```python
from build123d import *

# Parameters (mm, degrees)
SKETCH_R     = 2
PAD_DEPTH    = 10
PAD001_DEPTH = 10
PAD002_DEPTH = 10


with BuildPart() as part:
    # Sketch → Pad (new body)
    with BuildSketch(Plane.XY):
        with BuildLine():
            Line((-5, -25), (-5, 0))
            ThreePointArc((5, 0), (0, 5), (-5, 0))
            Line((5, 0), (5, -15))
            Line((5, -15), (70, -15))
            Line((70, -15), (70, 0))
            ThreePointArc((80, 0), (75, 5), (70, 0))
            Line((80, 0), (80, -25))
            Line((-5, -25), (80, -25))
        make_face()
        Circle(SKETCH_R, mode=Mode.SUBTRACT)
        with Locations((75, 0)):
            Circle(SKETCH_R, mode=Mode.SUBTRACT)
    extrude(amount=PAD_DEPTH)

    # Sketch001 (on Face1 of Pad) → Pad001 (join)
    with BuildSketch(Plane(origin=(-5, 0, 0), x_dir=(0, -1, 0), z_dir=(-1, 0, 0))):
        Polygon((25, 10), (-5, 61.961524), (-13.660254, 56.961524), (13.452995, 10), align=None)
    extrude(amount=-PAD001_DEPTH)

    # Sketch002 (on Face7 of Pad) → Pad002 (join)
    with BuildSketch(Plane.YZ.offset(80)):
        Polygon((-25, 10), (5, 61.961524), (13.660254, 56.961524), (-13.452995, 10), align=None)
    extrude(amount=-PAD002_DEPTH)


solid = part.part
```
The model under review builds one solid part; all positions refer to its coordinate system, in mm. A direction names the side the tool comes from. Round coordinates to 2 decimals unless told otherwise and drop trailing zeros. Order: outer loops, then holes, each group sorted by start corner. A loop starts at its lowest first (then second) coordinate and runs counter-clockwise, first axis right, second up. Notation, with made-up numbers: M -35.75,58 L 11.25,58 A15 ccw 11.25,86 Z; hole C 16,-39.75 d2. An arc over 180 degrees is marked long. Use a Markdown table: item, result.
1) Draft analysis for pull direction X (two halves, no side actions). For faces 6 (the face through (80, -7, 27)), 7 (the face through (5, -7, 29)), 8 (the face through (-0.07, -10.21, 35.62)), state which applies: released by +X, released by -X, zero draft, split by the parting line, or undercut.
Report:
| item | result |
|---|---|
| face 6 | released by +X |
| face 7 | undercut |
| face 8 | zero draft |
2) Consider section A-A (x = 75). Write out the cut boundary in (y, z), then the cut area to 3 significant figures.
Report:
| item | result |
|---|---|
| outline | M -25,0 L -2,0 L -2,10 L -13.45,10 L 13.66,56.96 L 5,61.96 L -25,10 Z; M 2,0 L 5,0 L 5,10 L 2,10 Z |
| area | 831 mm^2 |
3) Tool access review of faces 1 (the face through (70, -7, 29)), 2 (the face through (75.07, 0.293, 33.809)), 3 (the face through (38, -20, 10)), 4 (the face through (0, 5, 5)), 5 (the face through (37, -15, 5)): name each direction out of +Z, -Z, +X, -X, +Y, -Y from which nothing blocks a thin tool from reaching the whole face with its end or side.
Report:
| item | result |
|---|---|
| face 1 | +Z, +Y |
| face 2 | +X, -X, +Y |
| face 3 | +Z, +Y, -Y |
| face 4 | -Z, +Y |
| face 5 | +Z, -Z, +Y |
4) Insertion check: pin 1 (5 mm diameter, centred on x = 52.5, z = 4, fed in from +Y); pin 2 (8 mm diameter, centred on y = 7.5, z = 12, fed in from -X); pin 3 (2.5 mm diameter, centred on x = 0, y = 0, fed in from +Z). Each pin has a flat end and moves straight along its axis. Give the tip position at first contact, or say it passes through.
Report:
| item | result |
|---|---|
| pin 1 | y = -15 |
| pin 2 | x = -2.95 |
| pin 3 | z = 55.47 |
5) Consider section C-C (y = 8). Write out the cut boundary in (x, z), then the cut area to 3 significant figures.
Report:
| item | result |
|---|---|
| outline | M -5,47.16 L 5,47.16 L 5,60.23 L -5,60.23 Z; M 70,47.16 L 80,47.16 L 80,60.23 L 70,60.23 Z |
| area | 261 mm^2 |
6) Consider section D-D (y = -19.5). Write out the cut boundary in (x, z), then the cut area to 3 significant figures.
Report:
| item | result |
|---|---|
| outline | M -5,0 L 80,0 L 80,19.53 L 70,19.53 L 70,10 L 5,10 L 5,19.53 L -5,19.53 Z |
| area | 1,040 mm^2 |
7) Wall thickness on line 1 along Y through (x, z) = (0, 8); line 2 along Z through (x, y) = (10, -19); line 3 along X through (y, z) = (-8, 22): over which ranges is each line inside the solid? List them lowest first. Write a range as [from, to].
Report:
| item | result |
|---|---|
| line 1 | [-25, -2], [2, 5] |
| line 2 | [0, 10] |
| line 3 | [-5, 5], [70, 80] |
8) Consider section B-B (z = 42.5). Write out the cut boundary in (x, y), then the cut area to 3 significant figures.
Report:
| item | result |
|---|---|
| outline | M -5,-6.24 L 5,-6.24 L 5,5.31 L -5,5.31 Z; M 70,-6.24 L 80,-6.24 L 80,5.31 L 70,5.31 Z |
| area | 231 mm^2 |
